```python
from build123d import *

# Parameters (mm, degrees)
CROQUIS1_R              = 12.5
SALIENTE_EXTRUIR1_DEPTH = 23
CROQUIS2_R              = 3.5
SALIENTE_EXTRUIR2_DEPTH = 2
CROQUIS3_R              = 2
CORTAR_EXTRUIR2_DEPTH   = 6
CHAFL_N2_SIZE           = 0.2
CROQUIS4_W              = 0.1
CROQUIS4_H              = 0.1
CHAFL_N3_SIZE           = 0.2


with BuildPart() as part:
    # Croquis1 → Saliente-Extruir1 (new body)
    with BuildSketch(Plane.XY):
        Circle(CROQUIS1_R)
    extrude(amount=SALIENTE_EXTRUIR1_DEPTH)

    # Croquis2 → Saliente-Extruir2 (add)
    with BuildSketch(Plane.XY.offset(23)):
        Circle(CROQUIS2_R)
    extrude(amount=SALIENTE_EXTRUIR2_DEPTH)

    # Croquis3 → Cortar-Extruir2 (cut)
    with BuildSketch(Plane.XY.offset(25)):
        Circle(CROQUIS3_R)
    extrude(amount=-CORTAR_EXTRUIR2_DEPTH, mode=Mode.SUBTRACT)

    # Chaflán2
    chafl_n2_edges = [part.edges().sort_by_distance(p)[0] for p in [
        (-12.5, 0, 23),
    ]]
    chamfer(chafl_n2_edges, length=CHAFL_N2_SIZE)

    # Croquis4 → Cortar-Revolución1 (revolve, cut)
    with BuildSketch(Plane(origin=(0, 0, 0), x_dir=(1, 0, 0), z_dir=(0, 1, 0))):
        with Locations((-12.5, -4.6)):
            Rectangle(CROQUIS4_W, CROQUIS4_H)
        with Locations((-12.5, -18.4)):
            Rectangle(CROQUIS4_W, CROQUIS4_H)
    revolve(axis=Axis((0, 0, 0), (0, 0, 1)), mode=Mode.SUBTRACT)

    # Chaflán3
    chafl_n3_edges = [part.edges().sort_by_distance(p)[0] for p in [
        (-3.5, 0, 25),
    ]]
    chamfer(chafl_n3_edges, length=CHAFL_N3_SIZE)


solid = part.part
```
Can you work these out from the model? Positions are in its coordinate system, mm. A direction names the side the tool comes from. Coordinates: 2 decimals unless noted, no trailing zeros. Loops run counter-clockwise (first coordinate to the right, second up) from the corner with the lowest first, then second, coordinate; pieces in that order, holes last.
Item 1: Please list where these lines run through material, in increasing order: L1, parallel to Y at x = 0, z = 23.05; L2, parallel to Y at x = 0, z = 21; L3, parallel to Z at x = -8.25, y = -4.75.
Answers below:
L1: y = -3.5 to -2, 2 to 3.5
L2: y = -12.5 to -2, 2 to 12.5
L3: z = 0 to 23
Item 2: Which directions (+Z, -Z, +X, -X, +Y, -Y) give clear straight access to the entire face, cutting with the end or side of a thin tool? Please do faces 1 (the face through (11.923, 3.755, 11.404)), 2 (the face through (3, -3, 23)).
Answers below:
face 1: +Z, -Z
face 2: +Z
Item 3: I'm going to push flat-ended pins straight in: pin 1 (1.5 mm diameter, centred on y = 9, z = 13, fed in from +X); pin 2 (12 mm diameter, centred on x = 10, z = 19.5, fed in from -Y); pin 3 (3 mm diameter, centred on x = 0, y = 0, fed in from +Z). Where does each tip first touch, or does it pass through?
Answers below:
pin 1: stops at x = 9.39
pin 2: stops at y = -11.84
pin 3: stops at z = 19
Item 4: Suppose I cut it at C-C (z = 3). Please give me the cut outline in (x, y).
Answers below:
outline: circle Ø25 at (0, 0)
